CAD build for the part. Positions are in the model's coordinates, mm. A direction names the side the tool comes from. Give positions to 0.01 mm unless a question says otherwise; leave off trailing zeros. Write each loop counter-clockwise with the first axis right and the second up, starting at its lowest first coordinate (ties: lowest second). Pieces come first, ordered by that corner, then holes. Notation, with made-up numbers: (19, 35) - (26, 35) arc R12 cw to (26, 50) - close; hole circle Ø8 at (-24, -31). An arc over 180 degrees is marked (long way). Answer as a JSON object with one key per item and string values.
Autodesk Inventor part; units mm, degrees
ref_plane "Work Plane1" through (0, 0, -2.75) normal (0, 0, -1) x (-1, 0, 0)
ref_plane "YZ Plane" through (0, 0, 0) normal (1, 0, 0) x (0, 1, 0)
ref_plane "XZ Plane" through (0, 0, 0) normal (0, 1, 0) x (-1, 0, 0)
sketch "Sketch1" plane through (0, 0, 0) normal (0, 1, 0) x (-1, 0, 0)
  line L0 (0, 0) -> (0, -5.5)
  line L1 (0, -5.5) -> (4.0342, -5.5)
  line L2 (4.0342, -5.5) -> (10, -3.15)
  line L3 (10, -3.15) -> (10, -2.35)
  line L4 (10, -2.35) -> (4.0342, 0)
  line L5 (4.0342, 0) -> (0, 0)
  point P0 (10, -2.75)
  dimension "d0" = 43
  dimension "d2" = 0.8
  dimension "d3" = 10
  dimension "d4" = 5.5
revolve "Revolution1" add sketch "Sketch1" angle 360 about axis through (0, 0, 0) along (0, 0, -1)
sketch "Sketch2" plane through (0, 0, -5.5) normal (0, 0, -1) x (-1, 0, 0)
  circle A0 centre (0, 0) radius 4.0342
  circle A1 centre (0, 0) radius 1
  dimension "d6" = 2
extrude "Extrusion1" cut sketch "Sketch2" against normal through all contours A1
ref_plane "Work Plane1" through (0, 0, -2.75) normal (0, 0, -1) x (-1, 0, 0)
fillet "Fillet1" radius 0.5 2 edges at (10, 0, -2.35) (10, 0, -3.15)
split "Split1" plane through (0, 0, -2.75) removes the side toward (0, 0, 1)
sketch "Sketch3" plane through (0, 0, -5.5) normal (0, 0, -1) x (-1, 0, 0)
  circle A0 centre (0, 0) radius 1
  circle A1 centre (0, 0) radius 4.0342
extrude "Extrusion2" add sketch "Sketch3" along normal blind 2
chamfer "Chamfer1" distance 0.5 angle 45 1 edges at (4.0342, 0, -7.5)
properties part number "pritlacne_kolecko_polovina"
Item 1: Mould opens along Y. For faces 3 (the cylindrical face through (0, -1, -5)), 4 (the conical face through (0.95, 4.28, -5.36)), 5 (the flat face through (0, 2, -2.75)) say: +Y half, -Y half, draft (parallel to the pull), parting line (faces both ways), or undercut.
Entries:
{"face 3": "undercut", "face 4": "parting line", "face 5": "draft"}
Item 2: Which spindle directions (+Z, -Z, +X, -X, +Y, -Y) get a long thin tool onto all of the face, cutting with end or side? Do faces 1 (the flat face through (-1, -1, -7.5)), 2 (the cylindrical face through (0.87, 3.94, -6.24)). Say none if no direction does.
Entries:
{"face 1": "-Z, +X, -X, +Y, -Y", "face 2": "-Z"}
Item 3: Cut at A-A (z = -4.5). Give the cut face in (x, y).
Entries:
{"outline": "circle Ø13.15 at (0, 0); hole circle Ø2 at (0, 0)"}
Item 4: Probe line 1 (Y direction, x = 0, z = -5.55); line 2 (Y direction, x = 2.25, z = -3.05); line 3 (Z direction, x = 5, y = 7.5). List the from-to ranges inside material, lowest first. Write a range as from..to.
Entries:
{"line 1": "-4.03..-1, 1..4.03", "line 2": "-9.68..9.68", "line 3": "-3.54..-2.75"}
Item 5: Flat gauge pins, fed straight in: P1, Ø1.5, axis at x = -2.5, y = -5.5, coming from the -Z side; P2, Ø3, axis at x = -5.5, y = 3.5, coming from the -Z side; P3, Ø10, axis at x = -7, y = -5.5, coming from the -Z side. Where does each tip first touch, or does it go through?
Entries:
{"P1": "z = -5", "P2": "z = -5.11", "P3": "z = -7.13"}
